Here's the drawing with two shaded views (mm, measured from the low corner). I have some questions. A direction names the side the tool comes from. Round coordinates to 2 decimals unless told otherwise and drop trailing zeros. Loops run counter-clockwise (first coordinate to the right, second up) from the corner with the lowest first, then second, coordinate; pieces in that order, holes last.
(1) If I drill on line 1 along X through (y, z) = (1, 4.25); line 2 along Y through (x, z) = (12.5, 6.75); line 3 along Z through (x, y) = (13.5, 3.5), over which ranges is the centre line in solid material (lowest first)?
(2) I want a section at A-A on y = 7. Write out the boundary of the cut face in (x, z), plus the area to 3 significant figures.
(3) I want a section at C-C on x = 26. Write out the boundary of the cut face in (y, z), plus the area to 3 significant figures.
(4) Will these pins go through, and if not, where does the flat tip stop? pin 1 Ø3 at (x, y) = (8, 9.5) entering from +Z; pin 2 Ø4 at (x, z) = (12, 6.5) entering from -Y; pin 3 Ø3 at (x, z) = (26.5, 4) entering from +Y.
(5) Which directions (+Z, -Z, +X, -X, +Y, -Y) give clear straight access to the entire face, cutting with the end or side of a thin tool? Please do the marked faces 1 and 2.
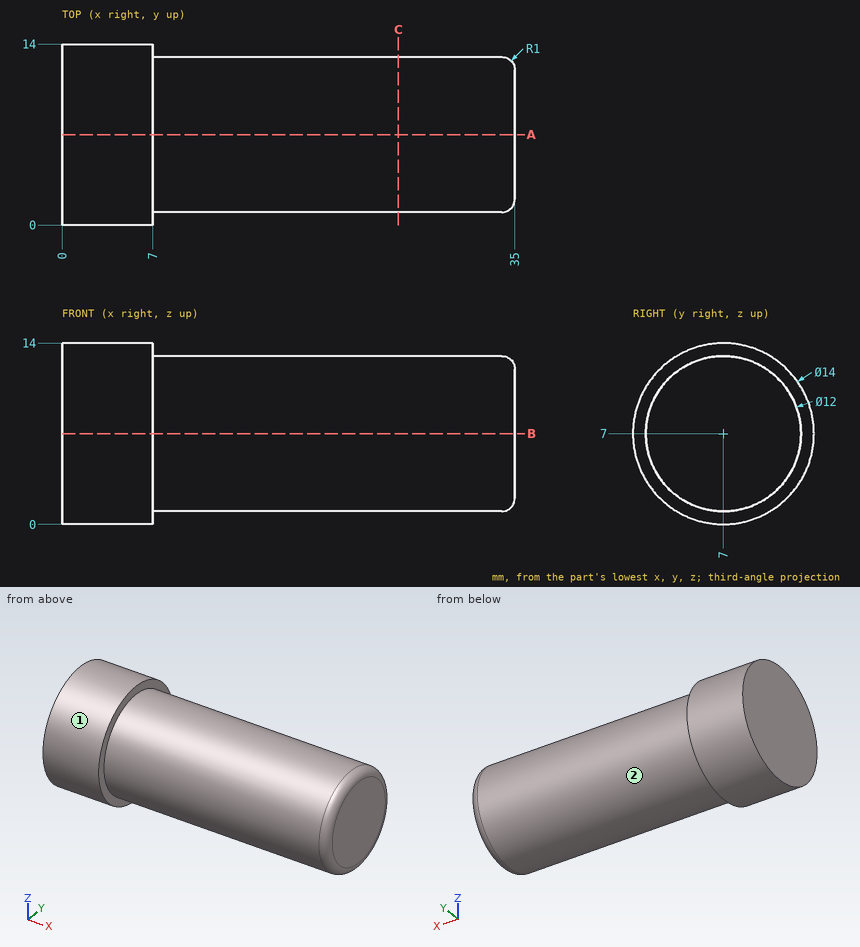
Filled sheet:
1. line 1: x = 0 to 7
1. line 2: y = 1.01 to 12.99
1. line 3: z = 2.13 to 11.87
2. outline: (0, 0) - (7, 0) - (7, 1) - (34, 1) arc R1 ccw to (35, 2) - (35, 12) arc R1 ccw to (34, 13) - (7, 13) - (7, 14) - (0, 14) - close
2. area: 434 mm2
3. outline: circle Ø12 at (7, 7)
3. area: 113 mm2
4. pin 1: stops at z = 13.86
4. pin 2: stops at y = 1
4. pin 3: stops at y = 12.81
5. face 1: +X, -X
5. face 2: +X
